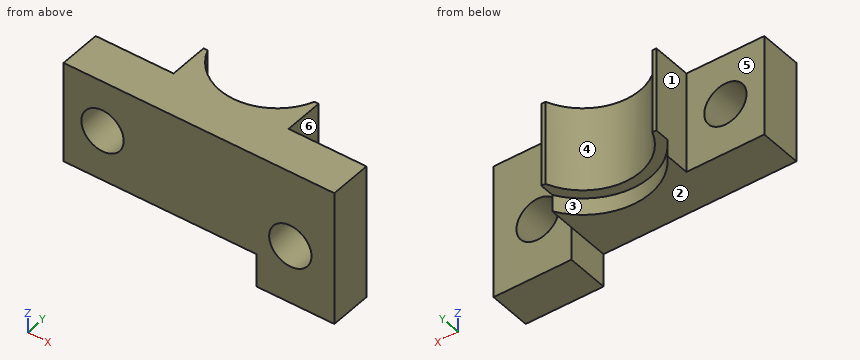
Autodesk Inventor part; units mm, degrees
ref_plane "YZ Plane" through (0, 0, 0) normal (1, 0, 0) x (0, 1, 0)
ref_plane "XZ Plane" through (0, 0, 0) normal (0, 1, 0) x (-1, 0, 0)
ref_plane "XY Plane" through (0, 0, 0) normal (0, 0, 1) x (1, 0, 0)
sketch "Sketch1" plane through (0, 0, 0) normal (0, 1, 0) x (-1, 0, 0)
  line L0 (0, 0) -> (20.32, 0)
  line L1 (20.32, 0) -> (20.32, 7.62)
  line L2 (20.32, 7.62) -> (0, 7.62)
  line L3 (0, 7.62) -> (0, 0)
  dimension "d0" = 20.32
  dimension "d1" = 7.62
extrude "Extrusion1" add sketch "Sketch1" along normal blind 3.175
sketch "Sketch2" plane through (0, 3.175, 0) normal (0, 1, 0) x (1, 0, 0)
  line L0 (0, 0) -> (-20.32, 0)
  line L1 (-20.32, 0) -> (-20.32, -7.62)
  line L2 (-20.32, -7.62) -> (0, -7.62)
  line L3 (-14.478, -7.62) -> (-5.842, -7.62)
  line L4 (-5.842, -7.62) -> (-5.842, 0)
  line L5 (-5.842, 0) -> (-14.478, 0)
  line L6 (-14.478, 0) -> (-14.478, -7.62)
  dimension "d4" = 8.636
  dimension "d5" = 5.842
extrude "Extrusion2" add sketch "Sketch2" along normal blind 7.112 contours L4 L2 L6 L0
sketch "Sketch3" plane through (-20.32, 0, 7.62) normal (0, 0, 1) x (1, 0, 0)
  line L0 (14.478, 3.175) -> (14.478, 10.287)
  line L1 (5.842, 10.287) -> (14.478, 10.287)
  circle A0 centre (10.16, 7.747) radius 4.318
  line L2 (5.842, 10.287) -> (14.478, 10.287)
  line L3 (14.478, 10.287) -> (14.478, 7.747)
  line L4 (14.478, 7.747) -> (5.842, 7.747)
  line L5 (5.842, 7.747) -> (5.842, 10.287)
  line L6 (5.842, 7.747) -> (14.478, 7.747)
  line L7 (14.478, 7.747) -> (14.478, 6.1492)
  line L8 (14.478, 6.1492) -> (5.842, 6.1492)
  line L9 (5.842, 6.1492) -> (5.842, 7.747)
  dimension "d8" = 8.636
  dimension "d9" = 2.54
extrude "Extrusion3" cut sketch "Sketch3" against normal up to surface (7.62 mm away)
sketch "Sketch5" plane through (0, 0, 0) normal (0, 0, -1) x (-1, 0, 0)
  arc A0 (6.1485, 6.1492) -> (14.1715, 6.1492) centre (10.16, 7.747) ccw
  circle A1 centre (10.16, 7.747) radius 5.08
  dimension "d21" = 10.16
extrude "Extrusion5" cut sketch "Sketch5" against normal blind 1.27
sketch "Sketch4" plane through (0, 0, 0) normal (0, -1, 0) x (1, 0, 0)
  line L0 (-20.32, 7.62) -> (0, 7.62)
  line L1 (-20.32, 0) -> (-20.32, 7.62)
  circle A0 centre (-17.399, 3.81) radius 1.5875
  circle A1 centre (-3.302, 1.8923) radius 1.5875
  dimension "d12" = 3.175
  dimension "d14" = 3.81
  dimension "d15" = 2.921
  dimension "d16" = 3.175
  dimension "d26" = 14.097
  dimension "d27" = 1.9177
extrude "Extrusion4" cut sketch "Sketch4" against normal up to next
sketch "Sketch6" plane through (0, 0, 0) normal (0, 0, -1) x (-1, 0, 0)
  line L0 (5.842, 3.175) -> (0, 3.175)
  line L1 (0, 3.175) -> (0, 0)
  line L2 (0, 0) -> (5.842, 0)
  line L3 (5.842, 0) -> (5.842, 3.175)
extrude "Extrusion6" add sketch "Sketch6" along normal blind 2.5
properties part number "Gbase 3"
Can you work these out from the model? Positions are in its coordinate system, mm. Face numbers are marked on the shaded views. A direction names the side the tool comes from. Give positions to 0.01 mm unless a question says otherwise; leave off trailing zeros. Order: outer loops, then holes, each group sorted by start corner. A loop starts at its lowest first (then second) coordinate and runs counter-clockwise, first axis right, second up. Notation, with made-up numbers: (55, 21) - (95, 21) arc R24 ccw to (95, 48) - close; hole circle Ø6 at (65.5, 16). An arc over 180 degrees is marked (long way). Use a Markdown table: item, result. Add a question column.
Q1. If we section it at B-B on y = 4.75: Write out the boundary of the cut face in (x, z).
Q2. If we section it at C-C on x = -18.75: Write out the boundary of the cut face in (y, z) (3 decimals), plus the area to 3 significant figures.
Q3. If we mould it in two halves opening along X, with no side actions, what happens to the marked faces 4, 5 and 6? For each: released by +X, released by -X, zero draft, split by the parting line, or undercut.
Q4. Please list where these lines run through material, in increasing order: line 1 along X through (y, z) = (0.5, 2.75); line 2 along Y through (x, z) = (-18, 5.75) (3 decimals); line 3 along Z through (x, y) = (-6, 1.5).
Q5. On a 3-axis mill with a long thin cutter (end or side, diameter ignored), from which of +Z, -Z, +X, -X, +Y, -Y can I reach the whole of each face in a straight line? I mean the marked faces 1, 2 and 3. Say none if no direction works.
Q6. I'm going to push flat-ended pins straight in: pin 1 (3 mm diameter, centred on x = -17.399, z = 3.81, fed in from +Y); pin 2 (1.5 mm diameter, centred on y = 5, z = 5, fed in from -X); pin 3 (1.5 mm diameter, centred on x = -10, y = 2.5, fed in from -Z); pin 4 (3 mm diameter, centred on x = -1.5, z = 3.5, fed in from +Y) (3 decimals). Where does each tip first touch, or does it pass through?
Q7. If we section it at D-D on y = 0.75: Write out the boundary of the cut face in (x, z) (1 decimal), plus the area to 3 significant figures.
Answers follow:
| question | item | result |
|---|---|---|
| 1 | outline | (-14.48, 0) - (-14.26, 0) - (-14.26, 1.27) - (-13.27, 1.27) - (-13.27, 7.62) - (-14.48, 7.62) - close; (-7.05, 1.27) - (-6.06, 1.27) - (-6.06, 0) - (-5.84, 0) - (-5.84, 7.62) - (-7.05, 7.62) - close |
| 2 | outline | (0, 0) - (3.175, 0) - (3.175, 2.976) - (0, 2.976) - close; (0, 4.644) - (3.175, 4.644) - (3.175, 7.62) - (0, 7.62) - close |
| 2 | area | 18.9 mm^2 |
| 3 | face 4 | undercut |
| 3 | face 5 | zero draft |
| 3 | face 6 | released by +X |
| 4 | line 1 | x = -20.32 to -18.58, -16.22 to -4.64, -1.97 to 0 |
| 4 | line 2 | y = 0 to 3.175 |
| 4 | line 3 | z = 0 to 7.62 |
| 5 | face 1 | +Z, -Z, -X, +Y |
| 5 | face 2 | -Z, -X, +Y, -Y |
| 5 | face 3 | -Z, +Y |
| 6 | pin 1 | passes through |
| 6 | pin 2 | stops at x = -14.48 |
| 6 | pin 3 | stops at z = 0 |
| 6 | pin 4 | stops at y = 3.175 |
| 7 | outline | (-20.3, 0) - (-5.8, 0) - (-5.8, -2.5) - (0, -2.5) - (0, 7.6) - (-20.3, 7.6) - close; hole circle Ø3.2 at (-17.4, 3.8); hole circle Ø3.2 at (-3.3, 1.9) |
| 7 | area | 154 mm^2 |
